Check sheet for the modelled part. Datum: model origin and axes. Units: mm. Face numbers are marked on the shaded views. Give positions to 0.01 mm unless a question says otherwise; leave off trailing zeros. Loops run counter-clockwise (first coordinate to the right, second up) from the corner with the lowest first, then second, coordinate; pieces in that order, holes last. Notation, with made-up numbers: (64, -14.75) -> (69, -14.75) arc R32 ccw to (69, 15.25) -> close; hole circle Ø2 at (36, 25.5). An arc over 180 degrees is marked (long way). Write each question's results on one line, items separated by ' | '. Start each with the question number.
Item 1: Scan lines: line 1 along Y through (x, z) = (-21.5, 11.25); line 2 along X through (y, z) = (-6.5, 19.5). Record each from-to range of solid material in increasing order.
Item 2: Mould release check, pull along Z, two halves, no side actions. Record for the marked faces 1, 2 and 3: pulls with the +Z half, pulls with the -Z half, needs draft (parallel to the pull), parting line crosses it, or undercut.
Item 3: Cross-section at A-A on y = -10. Enter the section's corners in (x, z).
Item 4: Cross-section at B-B on x = -30. Enter the section's corners in (y, z).
Item 5: Gauge pin test, flat end, axial feed: pin 1 Ø19.5 at (x, y) = (0, -20) entering from +Z. Record the tip position at first contact, or that the pin passes through.
from build123d import *

# Parameters (mm, degrees)
SKETCH1_W           = 80
SKETCH1_H           = 60
BOSS_EXTRUDE1_DEPTH = 30
SHELL1_START        = -39
SHELL1_OUTLINE_W    = 58
SHELL1_OUTLINE_H    = 28.99
SHELL1_DEPTH        = 78
CUT_EXTRUDE4_REACH  = 60.31
SKETCH2_R           = 7.5


# Read off the part's stored shape, not the designer's step: Shell1
with BuildPart() as part:
    # Sketch1 → Boss-Extrude1 (new body)
    with BuildSketch(Plane.XY):
        Rectangle(SKETCH1_W, SKETCH1_H)
    extrude(amount=BOSS_EXTRUDE1_DEPTH)

    # Shell1 outline → Shell1 (cut)
    with BuildSketch(Plane.YZ.offset(SHELL1_START)):
        with Locations((0, 15.495)):
            Rectangle(SHELL1_OUTLINE_W, SHELL1_OUTLINE_H)
    extrude(amount=SHELL1_DEPTH, mode=Mode.SUBTRACT)

    # Sketch2 → Cut-Extrude4 (cut, up to next)
    with BuildSketch(Plane.XY.offset(30), mode=Mode.PRIVATE) as cut_extrude4_sk1:
        with Locations((0, -20)):
            Circle(SKETCH2_R)
    cut_extrude4_tool1 = extrude(cut_extrude4_sk1.sketch, amount=-CUT_EXTRUDE4_REACH, mode=Mode.PRIVATE) & part.part
    add(cut_extrude4_tool1.solids().sort_by_distance((0, -20, 30))[0], mode=Mode.SUBTRACT)


solid = part.part
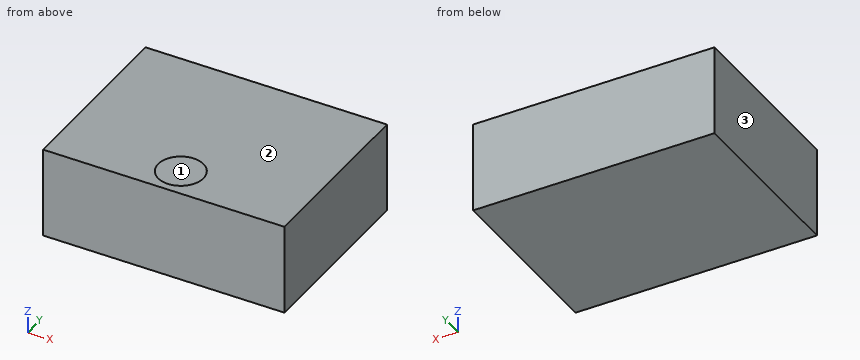
Answer sheet:
1) line 1: y = -30 to -29, 29 to 30 | line 2: x = -40 to -39, 39 to 40
2) face 1: undercut | face 2: pulls with the +Z half | face 3: needs draft
3) outline: (-40, 0) -> (40, 0) -> (40, 30) -> (-40, 30) -> close; hole (-39, 1) -> (39, 1) -> (39, 29.99) -> (-39, 29.99) -> close
4) outline: (-30, 0) -> (30, 0) -> (30, 30) -> (-30, 30) -> close; hole (-29, 1) -> (29, 1) -> (29, 29.99) -> (-29, 29.99) -> close
5) pin 1: stops at z = 30
